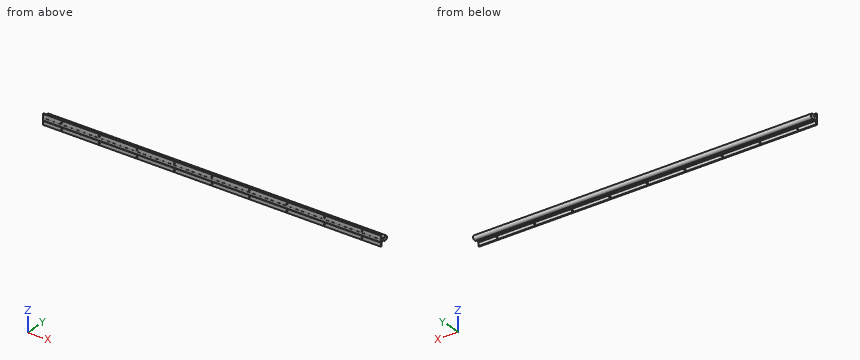
from build123d import *

# Parameters (mm, degrees)
EXTRUDE_1_DEPTH         = 1800
HOLE_WIZARD_6_6_6_6_1_D = 6.6
PATTERN_LINEAR_1_COUNT  = 9
PATTERN_LINEAR_1_PITCH  = 200


with BuildPart() as part:
    # 草图1 → 凸台-拉伸1 (new body)
    with BuildSketch(Plane(origin=(0, 0, 0), x_dir=(0, 0, -1), z_dir=(1, 0, 0))):
        with BuildLine():
            Line((38.023703704, 12.710240583), (38.023703704, 6.710240583))
            Line((38.023703704, 6.710240583), (18.023703704, 6.710240583))
            Line((18.023703704, 6.710240583), (16.823703704, 7.910240583))
            Line((16.823703704, 7.910240583), (4.223703704, 7.910240583))
            Line((4.223703704, 7.910240583), (3.023703704, 6.710240583))
            Line((3.023703704, 6.710240583), (-16.976296296, 6.710240583))
            Line((-16.976296296, 6.710240583), (-16.976296296, 12.710240583))
            Line((-16.976296296, 12.710240583), (1.023703704, 12.710240583))
            Line((1.023703704, 12.710240583), (1.023703704, 19.410240583))
            Line((1.023703704, 19.410240583), (2.593703704, 19.410240583))
            Line((2.593703704, 19.410240583), (5.975416608, 28.06708446))
            ThreePointArc((5.975416608, 28.06708446), (10.523703704, 52.210240583), (15.0719908, 28.06708446))
            Line((15.0719908, 28.06708446), (18.453703704, 19.410240583))
            Line((18.453703704, 19.410240583), (20.023703704, 19.410240583))
            Line((20.023703704, 19.410240583), (20.023703704, 12.710240583))
            Line((20.023703704, 12.710240583), (38.023703704, 12.710240583))
        make_face()
    extrude(amount=EXTRUDE_1_DEPTH)

    # Ø6.6 (6.6) 直径孔1 (through all)
    with Locations(Plane(origin=(100, 12.710240583, -28.023703704), x_dir=(0, 0, 1), z_dir=(0, 1, 0))):
        with Locations((0, 0), (35, 0)):
            hole_wizard_6_6_6_6_1 = Hole(HOLE_WIZARD_6_6_6_6_1_D / 2)

    # 阵列(线性)1: Ø6.6 (6.6) 直径孔1 ×9
    with Locations(*[(i * PATTERN_LINEAR_1_PITCH, 0, 0) for i in range(1, PATTERN_LINEAR_1_COUNT)]):
        add(hole_wizard_6_6_6_6_1, mode=Mode.SUBTRACT)


solid = part.part
Check sheet for the modelled part. Datum: model origin and axes. Units: mm. Round coordinates to 2 decimals unless told otherwise and drop trailing zeros. Loops run counter-clockwise (first coordinate to the right, second up) from the corner with the lowest first, then second, coordinate; pieces in that order, holes last. Notation, with made-up numbers: (-35.5, 16.25) - (-27.5, 16.25) arc R17 ccw to (-27.5, 24.25) - close; hole circle Ø9 at (38, 52). An arc over 180 degrees is marked (long way). Answer as CSV lines item,"result". Start each with the question number.
Item 1: Scan lines: line 1 (Z direction, x = 700, y = 8.15); line 2 (Y direction, x = 306, z = -12.5); line 3 (Z direction, x = 604.5, y = 18.5). Record each from-to range of solid material in increasing order. Write a range as [from, to].
Item 2: Depth check by flat-ended pin: P1, Ø6, axis at x = 1090.5, y = 34, coming from the -Z side; P2, Ø9, axis at x = 769.5, z = 5, coming from the +Y side; P3, Ø7.5, axis at x = 500, z = -28.02, coming from the +Y side; P4, Ø4, axis at x = 100, z = -28.02, coming from the -Y side. Enter the tip coordinate at first touch or a pass-through.
Item 3: Section check A-A (x = 633.5). Record the boundary of the cut face in (y, z).
Report:
1,line 1,"z = [-38.02, -31.32], [-24.72, 3.68], [10.28, 16.98]"
1,line 2,"y = [7.91, 52.05]"
1,line 3,"z = [-20.02, -1.02]"
2,P1,"stops at z = -22.73"
2,P2,"stops at y = 45.6"
2,P3,"stops at y = 12.71"
2,P4,"passes through"
3,outline,"(6.71, -38.02) - (12.71, -38.02) - (12.71, -20.02) - (19.41, -20.02) - (19.41, -18.45) - (28.07, -15.07) arc R12.5 ccw (long way) to (28.07, -5.98) - (19.41, -2.59) - (19.41, -1.02) - (12.71, -1.02) - (12.71, 16.98) - (6.71, 16.98) - (6.71, -3.02) - (7.91, -4.22) - (7.91, -16.82) - (6.71, -18.02) - close"
